CAD build for the part. Positions are in the model's coordinates, mm. A direction names the side the tool comes from. Give positions to 0.01 mm unless a question says otherwise; leave off trailing zeros. Order: outer loops, then holes, each group sorted by start corner. A loop starts at its lowest first (then second) coordinate and runs counter-clockwise, first axis right, second up. Notation, with made-up numbers: M 40.25,6 L 52.25,6 A30 ccw 52.25,31 Z; hole C 84.25,-22.5 d3. An arc over 180 degrees is marked long. Put each result on its own line as item: value. Start each with the question number.
1) Drill centre lines: line 1 (Z direction, x = 0, y = -3.15); line 2 (X direction, y = -3.9, z = 0.5); line 3 (X direction, y = -2.95, z = 4). Where is each one in solid material? Low to high. Write a range as [from, to].
2) Tool access for faces 1 (the face through (0, 0, 0)), 2 (the face through (-3.1, -3, 1)), 3 (the face through (0, -3, 6.4)), 4 (the face through (-3.1, -3, -6)): list every direction of +Z, -Z, +X, -X, +Y, -Y with a clear straight run to the whole face (end or side of a thin tool).
3) Cut at A-A (x = 5.75). Write the cut outline in (y, z), and give its area (4 significant figures).
4) Pin check, flat tips, straight feed: pin 1 (0.8 mm diameter, centred on x = 5.5, y = -3, fed in from -Z); pin 2 (1 mm diameter, centred on x = 5, z = -2.5, fed in from +Y); pin 3 (0.6 mm diameter, centred on x = 5.5, z = 0, fed in from -Y); pin 4 (3 mm diameter, centred on x = 1, y = -4, fed in from +Z). Stop position of each tip, or through.
5) Cut at D-D (x = 1.5). Write the cut outline in (y, z).
6) Cut at C-C (y = -4.95). Write the cut outline in (x, z).
7) Cut at B-B (z = 1). Write the cut outline in (x, y), and give its area (3 significant figures).
```python
from build123d import *

# Parameters (mm, degrees)
F0_W     = 6.2
F0_H     = 12.8
F1_DEPTH = 5.77
F2_W     = 0.375
F2_H     = 0.5
F2_W_2   = 0.75
F3_DEPTH = 4
F6_W     = 5.77
F6_H     = 12.66
F7_DEPTH = 0.3
F9_DEPTH = 0.3


# Not quite as in the source:
# - the program builds the solid bodies; features that only make, move or delete a surface that nothing else refers to are left out


with BuildPart() as f1:
    # F0 (on Front) → F1 (new body)
    with BuildSketch(Plane.XZ):
        Rectangle(F0_W, F0_H)
    extrude(amount=F1_DEPTH)

    # F2 (on face) → F3 (join)
    with BuildSketch(Plane.YZ.offset(3.1)):
        with Locations((-2.6975, 5.22)):
            Rectangle(F2_W, F2_H)
        with Locations((-3.0725, 5.22)):
            Rectangle(F2_W, F2_H)
        with Locations((-2.885, 0)):
            Rectangle(F2_W_2, F2_H)
        with Locations((-3.0725, -5.22)):
            Rectangle(F2_W, F2_H)
        with Locations((-2.6975, -5.22)):
            Rectangle(F2_W, F2_H)
    extrude(amount=F3_DEPTH)

    # F6 (on face) → F7 (join)
    with BuildSketch(Plane(origin=(-4.3378860758, 0, -1.2283157987), x_dir=(0, -1, 0), z_dir=(-0.962170457, 0, -0.2724481816))):
        with Locations((2.885, 1.7864348038)):
            Rectangle(F6_W, F6_H)
    extrude(amount=-F7_DEPTH)

    # F8 (on face) → F9 (cut, through all)
    with BuildSketch(Plane(origin=(-4.3378860758, 0, -1.2283157987), x_dir=(0, -1, 0), z_dir=(-0.962170457, 0, -0.2724481816))):
        Polygon((0, -4.5435651962), (1.6, 8.1164348038), (0, 8.1164348038), align=None)
        Polygon((4.17, 8.1164348038), (5.77, -4.5435651962), (5.77, 8.1164348038), align=None)
    extrude(amount=-F9_DEPTH, mode=Mode.SUBTRACT)


solid = f1.part
```
Solution:
1. line 1: [-6.4, 6.4]
1. line 2: [-4.83, -4.52], [-3.1, 3.1]
1. line 3: [-5.82, -5.51], [-3.1, 3.1]
2. face 1: +Z, -Z, +X, -X, +Y
2. face 2: +Z, +Y, -Y
2. face 3: +Z, +X, +Y, -Y
2. face 4: -Z, -X, +Y, -Y
3. outline: M -3.26,-5.47 L -2.51,-5.47 L -2.51,-4.97 L -3.26,-4.97 Z; M -3.26,-0.25 L -2.51,-0.25 L -2.51,0.25 L -3.26,0.25 Z; M -3.26,4.97 L -2.51,4.97 L -2.51,5.47 L -3.26,5.47 Z
3. area: 1.125 mm²
4. pin 1: z = -5.47
4. pin 2: through
4. pin 3: y = -3.26
4. pin 4: z = 6.4
5. outline: M -5.77,-6.4 L 0,-6.4 L 0,6.4 L -5.77,6.4 Z
6. outline: M -4.87,0.64 L -3.1,-5.6 L -3.1,-6.4 L 3.1,-6.4 L 3.1,6.4 L -3.1,6.4 L -3.1,-4.5 L -4.58,0.72 Z
7. outline: M -4.97,-4.9 L -4.66,-4.91 L -4.66,-0.86 L -4.97,-0.87 Z; M -3.1,-5.77 L 3.1,-5.77 L 3.1,0 L -3.1,0 Z
7. area: 37.0 mm²
